Geometry: final body of the model. Coordinates: model frame, mm. A direction names the side the tool comes from. Round coordinates to 2 decimals unless told otherwise and drop trailing zeros. Write each loop counter-clockwise with the first axis right and the second up, starting at its lowest first coordinate (ties: lowest second). Pieces come first, ordered by that corner, then holes. Notation, with made-up numbers: (51, 5.5) - (91, 5.5) arc R19 cw to (91, 31.5) - close; hole circle Ø4 at (76.5, 68). An arc over 180 degrees is marked (long way). Use a Markdown table: item, result. Add a question column.
```python
from build123d import *

# Parameters (mm, degrees)
BOSS_EXTRUDE1_DEPTH    = 3.175
SKETCH2_W              = 15
SKETCH2_H              = 55
BOSS_EXTRUDE2_DEPTH    = 5.5
CUT_EXTRUDE1_DEPTH     = 47.569840025
FILLET1_R              = 20
SKETCH6_W              = 31.616763165
SKETCH6_H              = 17.5
CUT_EXTRUDE3_DEPTH     = 50.489449633
BOSS_EXTRUDE4_DEPTH    = 3
FILLET3_R              = 5
SKETCH9_W              = 13
SKETCH9_H              = 1.5
CUT_EXTRUDE4_DEPTH     = 51.855333187
SPLIT1_SURFACE_1_BACK  = 62.685
SPLIT1_SURFACE_1_DEPTH = 125.37
SPLIT1_SURFACE_2_BACK  = 62.685
SPLIT1_SURFACE_2_DEPTH = 125.37
SKETCH12_W             = 4.85
SKETCH12_H             = 15
BOSS_EXTRUDE5_DEPTH    = 4


with BuildPart() as part:
    # Sketch1 → Boss-Extrude1 (new, symmetric)
    with BuildSketch(Plane(origin=(0, 0, 0), x_dir=(0, 0, -1), z_dir=(1, 0, 0))):
        Polygon((0, 0), (0, 23), (20, 23), (30, 6), (30, 0), align=None)
    extrude(amount=BOSS_EXTRUDE1_DEPTH, both=True)

    # Sketch2 → Boss-Extrude2 (add)
    with BuildSketch(Plane.XZ):
        with Locations((0, -15)):
            Rectangle(SKETCH2_W, SKETCH2_H)
    extrude(amount=-BOSS_EXTRUDE2_DEPTH)

    # Sketch3 → Cut-Extrude1 (cut, through all)
    with BuildSketch(Plane(origin=(0, 5.5, 0), x_dir=(1, 0, 0), z_dir=(0, 1, 0))):
        with BuildLine():
            Line((2.65, 45), (2.65, 35))
            ThreePointArc((2.65, 35), (0, 32.35), (-2.65, 35))
            Line((-2.65, 35), (-2.65, 45))
            ThreePointArc((-2.65, 45), (0, 47.65), (2.65, 45))
        make_face()
        with BuildLine():
            Line((2.65, -15), (2.65, -5))
            ThreePointArc((2.65, -5), (0, -2.35), (-2.65, -5))
            Line((-2.65, -5), (-2.65, -15))
            ThreePointArc((-2.65, -15), (0, -17.65), (2.65, -15))
        make_face()
    extrude(amount=-CUT_EXTRUDE1_DEPTH, mode=Mode.SUBTRACT)

    # Fillet1
    fillet1_edges = [part.edges().sort_by_distance(p)[0] for p in [
        (0, 23, -20),
    ]]
    fillet(fillet1_edges, radius=FILLET1_R)

    # Sketch6 → Cut-Extrude3 (cut, through all)
    with BuildSketch(Plane(origin=(3.175, 0, 0), x_dir=(0, 0, -1), z_dir=(1, 0, 0))):
        with Locations((15.808381583, 14.25)):
            Rectangle(SKETCH6_W, SKETCH6_H)
    extrude(amount=-CUT_EXTRUDE3_DEPTH, mode=Mode.SUBTRACT)

    # Sketch7 → Boss-Extrude4 (add, symmetric)
    with BuildSketch(Plane(origin=(0, 0, 0), x_dir=(0, 0, -1), z_dir=(1, 0, 0))):
        Polygon((0.5, 5.5), (0.5, 15.105993457), (24.253814646, 15.105993457), (24.253814646, 23.558754498), (33.902459411, 23.558754498), (33.902459411, 12.772125994), (29.5, 12.772125994), (29.5, 5.5), (15, 5.5), align=None)
    extrude(amount=BOSS_EXTRUDE4_DEPTH, both=True)

    # Fillet3
    # the kernel refuses this fillet: 5 mm, written as the material it adds along each edge
    with BuildSketch(Plane(origin=(3, 12.772125994, -29.5), x_dir=(0, -1, 0), z_dir=(-1, 0, 0))) as fillet3_piece_1:
        with BuildLine():
            CenterArc((4.964166118, -5), FILLET3_R, 90, 83.136284475)
            Line((0, -4.402459411), (0, 0))
            Line((0, 0), (4.964166118, 0))
        make_face()
    extrude(amount=6)
    with BuildSketch(Plane(origin=(3, 15.105993457, -24.253814646), x_dir=(0, 0, 1), z_dir=(-1, 0, 0))) as fillet3_piece_2:
        with BuildLine():
            CenterArc((FILLET3_R, FILLET3_R), FILLET3_R, 180, 90)
            Line((0, FILLET3_R), (0, 0))
            Line((0, 0), (FILLET3_R, 0))
        make_face()
    extrude(amount=6)
    # the kernel refuses this fillet: 5 mm, written as the material it takes off along each edge
    with BuildSketch(Plane(origin=(15.5, 15.105993457, -0.5), x_dir=(0, -1, 0), z_dir=(-1, 0, 0))) as fillet3_2_piece_1:
        with BuildLine():
            CenterArc((FILLET3_R, -FILLET3_R), FILLET3_R, 90, 90)
            Line((0, -FILLET3_R), (0, 0))
            Line((0, 0), (FILLET3_R, 0))
        make_face()
    extrude(amount=31, mode=Mode.SUBTRACT)

    # Sketch9 → Cut-Extrude4 (cut, through all)
    with BuildSketch(Plane(origin=(7.5, 0, 0), x_dir=(0, 0, -1), z_dir=(1, 0, 0))):
        with Locations((-6, 4.75)):
            Rectangle(SKETCH9_W, SKETCH9_H)
        with Locations((36, 4.75)):
            Rectangle(SKETCH9_W, SKETCH9_H)
    extrude(amount=-CUT_EXTRUDE4_DEPTH, mode=Mode.SUBTRACT)


with BuildPart() as body_2:
    # Split1: the piece behind the surface
    add(part.part)
    # Split1 surface: a surface, the sketch's curves swept straight by 125.37 mm
    with BuildLine(Plane(origin=(0, 0, -29.5), x_dir=(-1, 0, 0), z_dir=(0, 0, -1)).offset(-SPLIT1_SURFACE_1_BACK), mode=Mode.PRIVATE) as split1_surface_1_path:
        Line((-3, 7.807959877), (-3, 4))
        Line((-3, 4), (3, 4))
        Line((3, 4), (3, 7.807959877))
    split1_surface_1 = Shell.extrude(split1_surface_1_path.wire(), (0 * SPLIT1_SURFACE_1_DEPTH, 0 * SPLIT1_SURFACE_1_DEPTH, -1 * SPLIT1_SURFACE_1_DEPTH))
    split(bisect_by=split1_surface_1, keep=Keep.BOTTOM)

    # Sketch12 → Boss-Extrude5 (add)
    with BuildSketch(Plane(origin=(0, 4, 0), x_dir=(1, 0, 0), z_dir=(0, 1, 0))):
        with Locations((-5.075, 50)):
            Rectangle(SKETCH12_W, SKETCH12_H)
        with Locations((5.075, 50)):
            Rectangle(SKETCH12_W, SKETCH12_H)
        with Locations((-5.075, -20)):
            Rectangle(SKETCH12_W, SKETCH12_H)
        with Locations((5.075, -20)):
            Rectangle(SKETCH12_W, SKETCH12_H)
    extrude(amount=-BOSS_EXTRUDE5_DEPTH)


with BuildPart() as part_1:
    add(part.part)

    # Split1: split by a surface, the side it looks to stays
    # Split1 surface: a surface, the sketch's curves swept straight by 125.37 mm
    with BuildLine(Plane(origin=(0, 0, -29.5), x_dir=(-1, 0, 0), z_dir=(0, 0, -1)).offset(-SPLIT1_SURFACE_2_BACK), mode=Mode.PRIVATE) as split1_surface_2_path:
        Line((-3, 7.807959877), (-3, 4))
        Line((-3, 4), (3, 4))
        Line((3, 4), (3, 7.807959877))
    split1_surface_2 = Shell.extrude(split1_surface_2_path.wire(), (0 * SPLIT1_SURFACE_2_DEPTH, 0 * SPLIT1_SURFACE_2_DEPTH, -1 * SPLIT1_SURFACE_2_DEPTH))
    split(bisect_by=split1_surface_2, keep=Keep.TOP)


solid = body_2.part
```
1) Material intervals for L1, parallel to X at y = 4.5, z = -25; L2, parallel to X at y = 3.2, z = -49.5; L3, parallel to Y at x = 3.75, z = -39, sorted ascending. Write a range as from..to.
2) Section D-D, the plane z = -20. Return the cut outline in (x, y).
3) Set-up query: faces 1 (the flat face through (-2.65, 2, -46)), 2 (the flat face through (5, 5, -29.5)), 3 (the flat face through (3, 5, -15)), 4 (the flat face through (-2.65, 2, 16)). Return all of +Z, -Z, +X, -X, +Y, -Y with unobstructed straight access to the full face (end or side cutting, diameter ignored); none if empty.
4) Section C-C, the plane x = -6. Return the cut outline in (y, z), then the cut area to 4 significant figures.
5) Section B-B, the plane y = 2.9. Return the cut outline in (x, z).
6) Section A-A, the plane z = -36. Return the cut outline in (x, y), then the cut area to 3 significant figures.
7) Pin query (flat end, axial travel): P1, Ø4.5, axis at x = 0, z = -5, coming from the +Y side; P2, Ø1.5, axis at x = 5.5, y = 5, coming from the +Z side. Return the tip coordinate at first contact, or that it passes through.
8) Draft query along X for faces 5 (the flat face through (7.5, 2, -16)), 6 (the flat face through (-5, 2, 27.5)), 7 (the cylindrical face through (0.06, 2.03, 2.35)). Return one class per face: released by +X, released by -X, zero draft, split by the parting line, or undercut.
Output values:
| question | item | result |
|---|---|---|
| 1 | L1 | x = -7.5..-3, 3..7.5 |
| 1 | L2 | x = -7.5..-2.65, 2.65..7.5 |
| 1 | L3 | y = 0..4 |
| 2 | outline | (-7.5, 0) - (7.5, 0) - (7.5, 5.5) - (3, 5.5) - (3, 4) - (-3, 4) - (-3, 5.5) - (-7.5, 5.5) - close |
| 3 | face 1 | -Z, +Y, -Y |
| 3 | face 2 | -Z, +X, -X, +Y |
| 3 | face 3 | +Z, -Z, +Y |
| 3 | face 4 | +Z, +Y, -Y |
| 4 | outline | (0, -57.5) - (4, -57.5) - (4, -29.5) - (5.5, -29.5) - (5.5, -0.5) - (4, -0.5) - (4, 27.5) - (0, 27.5) - close |
| 4 | area | 383.5 mm^2 |
| 5 | outline | (-7.5, -57.5) - (-2.65, -57.5) - (-2.65, -35) arc R2.65 cw to (2.65, -35) - (2.65, -57.5) - (7.5, -57.5) - (7.5, 27.5) - (2.65, 27.5) - (2.65, 5) arc R2.65 cw to (-2.65, 5) - (-2.65, 27.5) - (-7.5, 27.5) - close |
| 6 | outline | (-7.5, 0) - (-2.65, 0) - (-2.65, 4) - (-7.5, 4) - close; (2.65, 0) - (7.5, 0) - (7.5, 4) - (2.65, 4) - close |
| 6 | area | 38.8 mm^2 |
| 7 | P1 | stops at y = 4 |
| 7 | P2 | stops at z = -0.5 |
| 8 | face 5 | released by +X |
| 8 | face 6 | zero draft |
| 8 | face 7 | undercut |
